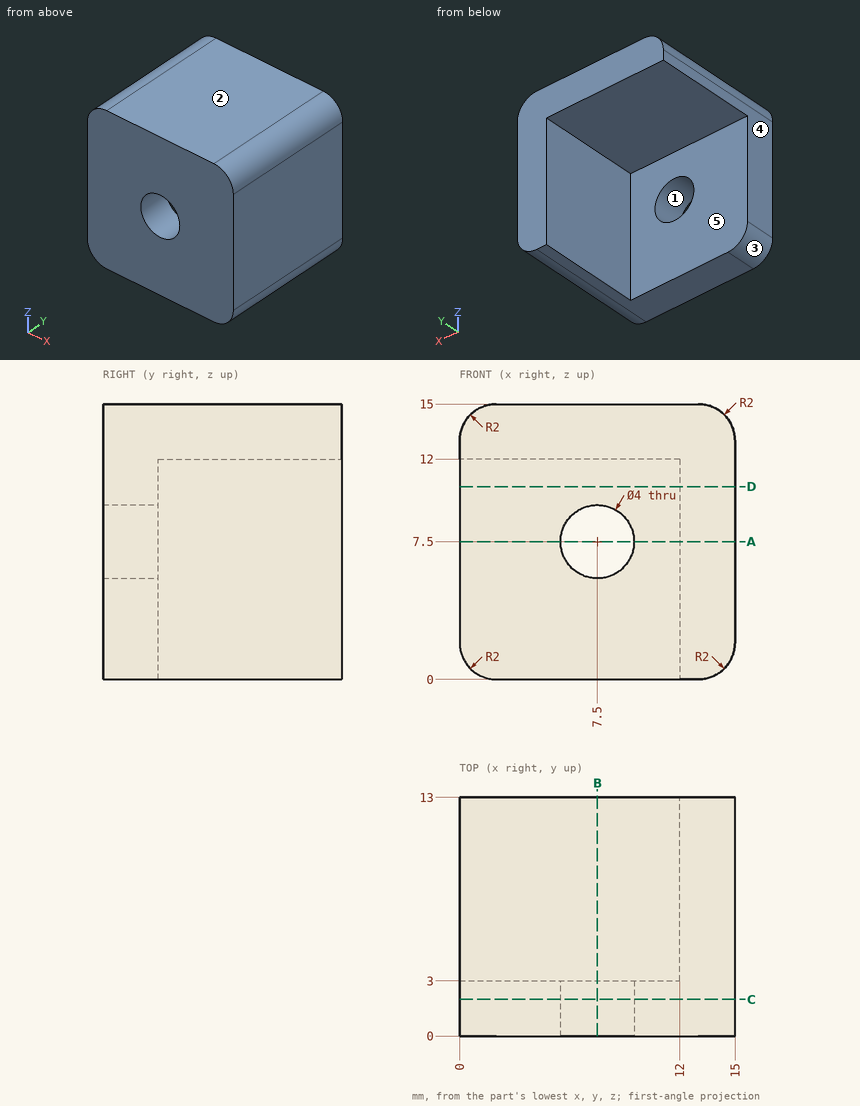
Can you work these out from the drawing? Everything is in mm from the part's minimum corner. A direction names the side the tool comes from. Give positions to 0.01 mm unless a question says otherwise; leave off trailing zeros. Order: outer loops, then holes, each group sorted by start corner. A loop starts at its lowest first (then second) coordinate and runs counter-clockwise, first axis right, second up. Notation, with made-up numbers: M 10.25,-3.5 L 39.25,-3.5 A14 cw 39.25,13.5 Z; hole C 38.25,46 d3. An arc over 180 degrees is marked long. Use a Markdown table: item, result. Add a question column.
Item 1: If I drill on L1, parallel to X at y = 0.8, z = 7.5; L2, parallel to Z at x = 11.25, y = 3.5, over which ranges is the centre line in solid material (lowest first)? Write a range as [from, to].
Item 2: We'd pull the mould along X, two halves only. Please class the marked faces 1, 2 and 3: +X half, -X half, draft (parallel to the pull), parting line (faces both ways), or undercut.
Item 3: For the marked faces 4 and 5, which set-ups out of +Z, -Z, +X, -X, +Y, -Y let a thin tool reach every point of the face, with its end or its side?
Item 4: Suppose I cut it at B-B (x = 7.5). List the corners of the cut face in (y, z) for me.
Item 5: Suppose I cut it at D-D (z = 10.5). List the corners of the cut face in (x, y) for me, then the cut area to 3 significant figures.
Item 6: Will these pins go through, and if not, where does the flat tip stop? pin 1 (2 mm diameter, centred on y = 9.5, z = 10.5, fed in from -X); pin 2 (1 mm diameter, centred on x = 2, y = 8.5, fed in from -Z); pin 3 (3.5 mm diameter, centred on x = 6, z = 7.5, fed in from +Y).
Item 7: Suppose I cut it at A-A (z = 7.5). List the corners of the cut face in (x, y) for me, then the cut area to 3 significant figures.
Item 8: Suppose I cut it at C-C (y = 2). List the corners of the cut face in (x, z) for me.
Answer sheet:
| question | item | result |
|---|---|---|
| 1 | L1 | x = [0, 5.5], [9.5, 15] |
| 1 | L2 | z = [12, 15] |
| 2 | face 1 | undercut |
| 2 | face 2 | draft |
| 2 | face 3 | -X half |
| 3 | face 4 | +Z, -Z, -X, +Y, -Y |
| 3 | face 5 | -Z, -X, +Y |
| 4 | outline | M 0,0 L 3,0 L 3,5.5 L 0,5.5 Z; M 0,9.5 L 3,9.5 L 3,12 L 13,12 L 13,15 L 0,15 Z |
| 5 | outline | M 0,0 L 15,0 L 15,13 L 12,13 L 12,3 L 0,3 Z |
| 5 | area | 75.0 mm² |
| 6 | pin 1 | stops at x = 12 |
| 6 | pin 2 | stops at z = 12 |
| 6 | pin 3 | stops at y = 3 |
| 7 | outline | M 0,0 L 5.5,0 L 5.5,3 L 0,3 Z; M 9.5,0 L 15,0 L 15,13 L 12,13 L 12,3 L 9.5,3 Z |
| 7 | area | 63.0 mm² |
| 8 | outline | M 0,2 A2 ccw 2,0 L 13,0 A2 ccw 15,2 L 15,13 A2 ccw 13,15 L 2,15 A2 ccw 0,13 Z; hole C 7.5,7.5 d4 |
